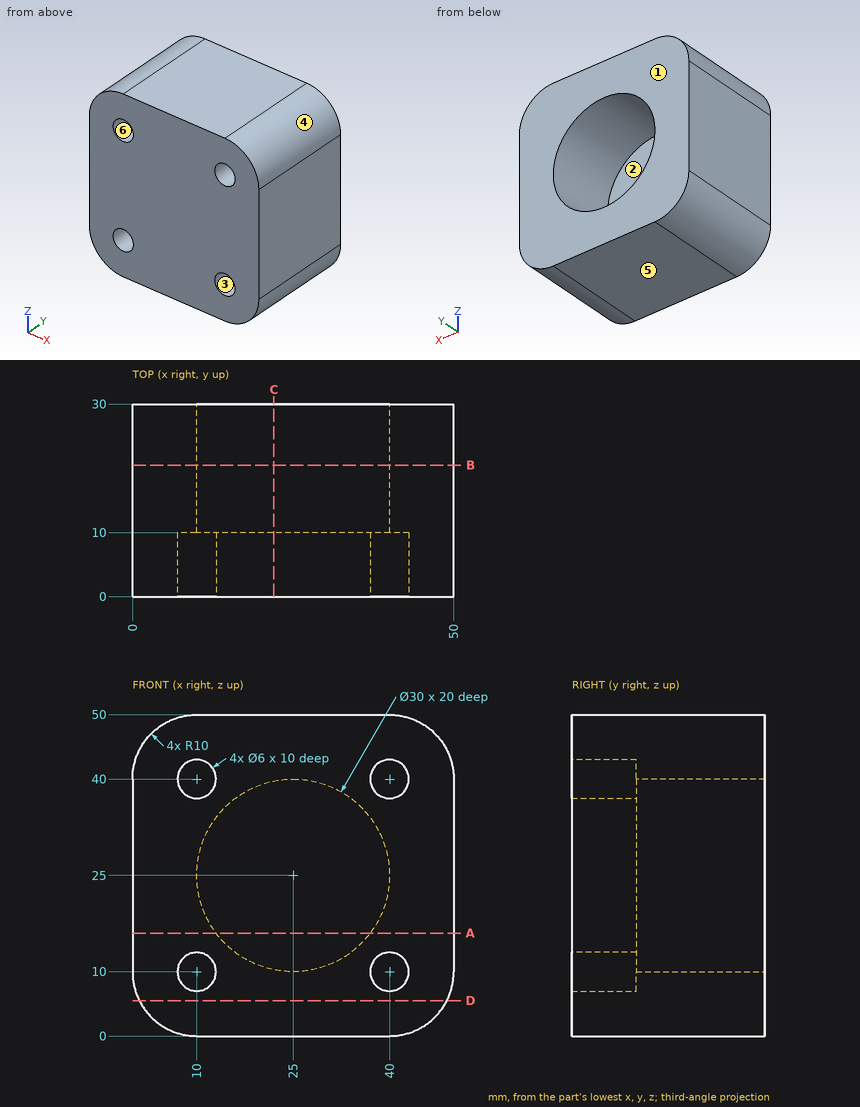
Can you work these out from the drawing? Everything is in mm from the part's minimum corner. A direction names the side the tool comes from. Give positions to 0.01 mm unless a question says otherwise; leave off trailing zeros. Loops run counter-clockwise (first coordinate to the right, second up) from the corner with the lowest first, then second, coordinate; pieces in that order, holes last. Notation, with made-up numbers: (6.25, 15) -> (27.25, 15) arc R25 cw to (27.25, 37) -> close; hole circle Ø2 at (44, 40). An arc over 180 degrees is marked (long way). Write item = value, one per line.
1) Will these pins go through, and if not, where does the flat tip stop? pin 1 (6 mm diameter, centred on x = 21.5, z = 22.5, fed in from +Y); pin 2 (6 mm diameter, centred on y = 19, z = 5, fed in from +X); pin 3 (1.5 mm diameter, centred on y = 16, z = 41, fed in from +X).
Check result:
pin_1 = 10
pin_2 = 49.8
pin_3 = 50
2) Suppose I cut it at C-C on x = 22. Write out the boundary of the cut face in (y, z).
Check result:
outline = (0, 0) -> (30, 0) -> (30, 10.3) -> (10, 10.3) -> (10, 39.7) -> (30, 39.7) -> (30, 50) -> (0, 50) -> close
3) Suppose I cut it at A-A on z = 16. Write out the boundary of the cut face in (x, y).
Check result:
outline = (0, 0) -> (50, 0) -> (50, 30) -> (37, 30) -> (37, 10) -> (13, 10) -> (13, 30) -> (0, 30) -> close
4) Thinking about a two-plate mould opening in Z: for the marked faces 4, 5 and 6, which applies, released by +Z, released by -Z, zero draft, split by the parting line, or undercut?
Check result:
face_4 = released by +Z
face_5 = released by -Z
face_6 = undercut
5) Suppose I cut it at D-D on z = 5.5. Write out the boundary of the cut face in (x, y), then the cut area to 3 significant figures.
Check result:
outline = (1.07, 0) -> (48.93, 0) -> (48.93, 30) -> (1.07, 30) -> close
area = 1,440 mm2
6) Suppose I cut it at B-B on y = 20.5. Write out the boundary of the cut face in (x, z), then the cut area to 3 significant figures.
Check result:
outline = (0, 10) arc R10 ccw to (10, 0) -> (40, 0) arc R10 ccw to (50, 10) -> (50, 40) arc R10 ccw to (40, 50) -> (10, 50) arc R10 ccw to (0, 40) -> close; hole circle Ø30 at (25, 25)
area = 1,710 mm2
7) I need wall thicknesses on L1, parallel to X at y = 4.75, z = 10; L2, parallel to X at y = 23, z = 25; L3, parallel to Y at x = 20, z = 21.5. Which ranges of each line are inside material? Lowest first, please. Write a range as from..to.
Check result:
L1 = 0..7, 13..37, 43..50
L2 = 0..10, 40..50
L3 = 0..10
8) For the marked faces 1, 2 and 3, which set-ups out of +Z, -Z, +X, -X, +Y, -Y let a thin tool reach every point of the face, with its end or its side?
Check result:
face_1 = +Z, -Z, +X, -X, +Y
face_2 = +Y
face_3 = -Y
